Autodesk Inventor part; units mm, degrees
ref_plane "Plano de trabajo1" through (0, 9, 0) normal (0, 1, 0) x (-1, 0, 0)
ref_plane "YZ Plane" through (0, 0, 0) normal (1, 0, 0) x (0, 1, 0)
ref_plane "XY Plane" through (0, 0, 0) normal (0, 0, 1) x (1, 0, 0)
sketch "Boceto1" plane through (0, 0, 0) normal (1, 0, 0) x (0, 1, 0)
  line L0 (0, 0) -> (18, 0)
  line L1 (0, 0) -> (0, -4.8)
  line L2 (18, 0) -> (23, 0)
  line L3 (18, 0) -> (18, -3.8)
  line L4 (0, 0) -> (-5, 0)
  line L5 (-5, 0) -> (-5, 3.8)
  dimension "d0" = 18
  dimension "d1" = 4.8
  dimension "d2" = 5
  dimension "d4" = 3.8
  dimension "d5" = 5
  dimension "d6" = 3.8
sketch "Boceto4" plane through (0, 0, 0) normal (0, 1, 0) x (-1, 0, 0)
  circle A0 centre (0, 0) radius 2.4
  dimension "d10" = 4.8
sweep "Barrido1" add profiles "Boceto4" path "Boceto1" path curves L0
ref_plane "Plano de trabajo1" through (0, 9, 0) normal (0, 1, 0) x (-1, 0, 0)
sketch "Boceto5" plane through (0, 9, 0) normal (0, 1, 0) x (-1, 0, 0)
  circle A0 centre (0, 0) radius 1.9
  dimension "d14" = 3.8
extrude "Extrusión1" add sketch "Boceto5" along normal mid plane 28
Here's how the part is built. I have some questions about the finished solid (model axes, mm). A direction names the side the tool comes from. Coordinates: 2 decimals unless noted, no trailing zeros. Loops run counter-clockwise (first coordinate to the right, second up) from the corner with the lowest first, then second, coordinate; pieces in that order, holes last. Notation, with made-up numbers: (52, 80.25) -> (61, 80.25) arc R25 cw to (61, 111.25) -> close; hole circle Ø9 at (-24.5, 31.5). An arc over 180 degrees is marked (long way). Return JSON: item names as keys, results as strings.
1) For faces 1 (the face through (1, 0, 2)), 2 (the face through (1.9, 20.46, -0.08)), 3 (the face through (0, 23, 0)), which set-ups out of +Z, -Z, +X, -X, +Y, -Y let a thin tool reach every point of the face, with its end or its side?
Results below:
{"face 1": "-Y", "face 2": "+Y", "face 3": "+Z, -Z, +X, -X, +Y"}
2) If we section it at A-A, the plane x = 0: Write out the boundary of the cut face in (y, z).
Results below:
{"outline": "(-5, -1.9) -> (0, -1.9) -> (0, -2.4) -> (18, -2.4) -> (18, -1.9) -> (23, -1.9) -> (23, 1.9) -> (18, 1.9) -> (18, 2.4) -> (0, 2.4) -> (0, 1.9) -> (-5, 1.9) -> close"}
3) I need wall thicknesses on line 1 (Y direction, x = -1.7, z = 1); line 2 (X direction, y = 4.5, z = 0.15). Which ranges of each line are inside material? Lowest first, please. Write a range as from..to.
Results below:
{"line 1": "0..18", "line 2": "-2.4..2.4"}
4) If we section it at B-B, the plane z = 0: Write out the boundary of the cut face in (x, y).
Results below:
{"outline": "(-2.4, 0) -> (-1.9, 0) -> (-1.9, -5) -> (1.9, -5) -> (1.9, 0) -> (2.4, 0) -> (2.4, 18) -> (1.9, 18) -> (1.9, 23) -> (-1.9, 23) -> (-1.9, 18) -> (-2.4, 18) -> close"}
5) If we section it at D-D, the plane y = 5.5: Write out the boundary of the cut face in (x, z).
Results below:
{"outline": "circle Ø4.8 at (0, 0)"}
6) If we section it at C-C, the plane y = -2.25: Write out the boundary of the cut face in (x, z), then the cut area to 3 significant figures.
Results below:
{"outline": "circle Ø3.8 at (0, 0)", "area": "11.3 mm²"}
7) Will this pin go through, and if not, where does the flat tip stop? pin 1 (1 mm diameter, centred on x = 1.5, y = 19.5, fed in from -Z).
Results below:
{"pin 1": "z = -1.62"}
